from build123d import *

# Parameters (mm, degrees)
CUT_EXTRUDE1_DEPTH = 1
SKETCH4_R          = 2.309401077
CUT_EXTRUDE2_DEPTH = 0.5
CUT_EXTRUDE2_TAPER = 45


with BuildPart() as part:
    # Sketch2 → Revolve1 (revolve)
    with BuildSketch(Plane(origin=(0, 0, 0), x_dir=(0, 0, -1), z_dir=(1, 0, 0))):
        Polygon((-6.25, 4.25), (-1.75, 4.25), (-1.5, 4), (-1.5, 2.5), (5.7, 2.5), (6.5, 1.7), (6.5, 0), (-6.5, 0), (-6.5, 4), align=None)
    revolve(axis=Axis((0, 0, -6.5), (0, 0, 1)))

    # Sketch3 → Cut-Extrude1 (cut)
    with BuildSketch(Plane.XY.offset(6.5)):
        Polygon((1.154700538, 2), (-1.154700538, 2), (-2.309401077, 0), (-1.154700538, -2), (1.154700538, -2), (2.309401077, 0), align=None)
    extrude(amount=-CUT_EXTRUDE1_DEPTH, mode=Mode.SUBTRACT)

    # Sketch4 → Cut-Extrude2 (cut)
    with BuildSketch(Plane.XY.offset(6.5)):
        Circle(SKETCH4_R)
    extrude(amount=-CUT_EXTRUDE2_DEPTH, taper=CUT_EXTRUDE2_TAPER, mode=Mode.SUBTRACT)


solid = part.part
Build history of the part. All positions in model axes, mm. A direction names the side the tool comes from. Round coordinates to 2 decimals unless told otherwise and drop trailing zeros. Loops run counter-clockwise (first coordinate to the right, second up) from the corner with the lowest first, then second, coordinate; pieces in that order, holes last. Notation, with made-up numbers: (31, 14) -> (48, 14) arc R16 cw to (48, 19) -> close; hole circle Ø4 at (75.25, 56.5). An arc over 180 degrees is marked (long way). Answer in a Markdown table with one row per item.
Item 1: Mould opens along Y. For faces 4 (the cylindrical face through (-3.584, 2.285, 3.968)), 5 (the flat face through (-1.724, 1.014, 5.896)), 6 (the flat face through (0, 0, -6.5)) say: +Y half, -Y half, draft (parallel to the pull), parting line (faces both ways), or undercut.
Answers below:
| item | result |
|---|---|
| face 4 | parting line |
| face 5 | undercut |
| face 6 | draft |
Item 2: Drill centre lines: L1, parallel to Z at x = 2, y = -2.25; L2, parallel to X at y = 0, z = -4.75; L3, parallel to Y at x = -1.5, z = -5.5. Where is each one in solid material? Low to high. Write a range as [from, to].
Answers below:
| item | result |
|---|---|
| L1 | z = [1.5, 6.5] |
| L2 | x = [-2.5, 2.5] |
| L3 | y = [-2, 2] |
Item 3: Saw through at B-B (x = 0). Write the cut outline in (y, z), and give its area (3 significant figures).
Answers below:
| item | result |
|---|---|
| outline | (-4.25, 1.75) -> (-4, 1.5) -> (-2.5, 1.5) -> (-2.5, -5.7) -> (-1.7, -6.5) -> (1.7, -6.5) -> (2.5, -5.7) -> (2.5, 1.5) -> (4, 1.5) -> (4.25, 1.75) -> (4.25, 6.25) -> (4, 6.5) -> (2.31, 6.5) -> (2, 6.19) -> (2, 5.5) -> (-2, 5.5) -> (-2, 6.19) -> (-2.31, 6.5) -> (-4, 6.5) -> (-4.25, 6.25) -> close |
| area | 77.6 mm² |
Item 4: Which spindle directions (+Z, -Z, +X, -X, +Y, -Y) get a long thin tool onto all of the face, cutting with end or side? Do faces 1 (the flat face through (2, -2, 6.5)), 2 (the conical face through (1.856, -1.09, 6.343)), 3 (the flat face through (-2, 2, 1.5)). Say none if no direction does.
Answers below:
| item | result |
|---|---|
| face 1 | +Z, +X, -X, +Y, -Y |
| face 2 | +Z |
| face 3 | -Z |
Item 5: Saw through at C-C (z = -0.25). Write the cut outline in (x, y).
Answers below:
| item | result |
|---|---|
| outline | circle Ø5 at (0, 0) |
Item 6: Pin check, flat tips, straight feed: pin 1 (1.5 mm diameter, centred on x = -1.5, z = -0.5, fed in from +Y); pin 2 (3 mm diameter, centred on x = -0.5, z = -2, fed in from +Y); pin 3 (3 mm diameter, centred on y = -2.5, z = -2.5, fed in from -X). Stop position of each tip, or through.
Answers below:
| item | result |
|---|---|
| pin 1 | stops at y = 2.38 |
| pin 2 | stops at y = 2.5 |
| pin 3 | stops at x = -2.29 |
Item 7: Saw through at A-A (z = 5.75). Write the cut outline in (x, y).
Answers below:
| item | result |
|---|---|
| outline | circle Ø8.5 at (0, 0); hole (-2.31, 0) -> (-1.15, -2) -> (1.15, -2) -> (2.31, 0) -> (1.15, 2) -> (-1.15, 2) -> close |
